from build123d import *

# Parameters (mm, degrees)
SKETCH1_R           = 5
BOSS_EXTRUDE1_DEPTH = 10
SKETCH3_W           = 10
SKETCH3_H           = 4.789047851
BOSS_EXTRUDE2_DEPTH = 15
SKETCH4_W           = 15
SKETCH4_H           = 4.789047851
BOSS_EXTRUDE3_DEPTH = 30
CUT_EXTRUDE1_REACH  = 9.289
SKETCH5_R           = 1.5


with BuildPart() as part:
    # Sketch1 → Boss-Extrude1 (new body)
    with BuildSketch(Plane.XY):
        with BuildLine():
            Line((0, 10), (-35, 7.5))
            Line((-35, 7.5), (-35, -7.5))
            Line((-35, -7.5), (0, -10))
            ThreePointArc((0, -10), (10, 0), (0, 10))
        make_face()
        Circle(SKETCH1_R, mode=Mode.SUBTRACT)
    extrude(amount=BOSS_EXTRUDE1_DEPTH)

    # Sketch3 → Boss-Extrude2 (add)
    with BuildSketch(Plane.ZY.offset(35)):
        with Locations((5, -5.105476075)):
            Rectangle(SKETCH3_W, SKETCH3_H)
    extrude(amount=BOSS_EXTRUDE2_DEPTH)

    # Sketch4 → Boss-Extrude3 (add)
    with BuildSketch(Plane(origin=(0, 0, 0), x_dir=(-1, 0, 0), z_dir=(0, 0, -1))):
        with Locations((42.5, -5.105476075)):
            Rectangle(SKETCH4_W, SKETCH4_H)
    extrude(amount=BOSS_EXTRUDE3_DEPTH)

    # Sketch5 → Cut-Extrude1 (cut, up to next)
    with BuildSketch(Plane(origin=(0, -2.710952149, 0), x_dir=(1, 0, 0), z_dir=(0, 1, 0)), mode=Mode.PRIVATE) as cut_extrude1_sk1:
        with Locations((-39, 2.273461037)):
            Circle(SKETCH5_R)
    cut_extrude1_tool1 = extrude(cut_extrude1_sk1.sketch, amount=-CUT_EXTRUDE1_REACH, mode=Mode.PRIVATE) & part.part
    add(cut_extrude1_tool1.solids().sort_by_distance((-39, -2.710952, -2.273461))[0], mode=Mode.SUBTRACT)
    # Sketch5 → Cut-Extrude1 (cut, up to next)
    with BuildSketch(Plane(origin=(0, -2.710952149, 0), x_dir=(1, 0, 0), z_dir=(0, 1, 0)), mode=Mode.PRIVATE) as cut_extrude1_sk2:
        with Locations((-39, 14.273461037)):
            Circle(SKETCH5_R)
    cut_extrude1_tool2 = extrude(cut_extrude1_sk2.sketch, amount=-CUT_EXTRUDE1_REACH, mode=Mode.PRIVATE) & part.part
    add(cut_extrude1_tool2.solids().sort_by_distance((-39, -2.710952, -14.273461))[0], mode=Mode.SUBTRACT)


solid = part.part
The listing builds one solid part. Answer for the finished solid, in the listing's coordinates (mm). A direction names the side the tool comes from. Round coordinates to 2 decimals unless told otherwise and drop trailing zeros. Write each loop counter-clockwise with the first axis right and the second up, starting at its lowest first coordinate (ties: lowest second). Pieces come first, ordered by that corner, then holes. Notation, with made-up numbers: M -3,-15 L 47,-15 A19 ccw 47,-8 Z; hole C 89,-20.5 d1. An arc over 180 degrees is marked long. Write each question's results on one line, items separated by ' | '. Start each with the question number.
Item 1: Find section A-A on y = 0. Write down the section's boundary in (x, z).
Item 2: Find section B-B on x = -39. Write down the section's boundary in (y, z).
Item 3: Which of the six approach directions +Z, -Z, +X, -X, +Y, -Y give full straight-line access (tool end or side, diameter ignored) to faces 1 (the flat face through (-42, -7.5, -10)), 2 (the flat face through (-35, 2, 5)), 3 (the flat face through (-35, -5, -15))?
Item 4: Straight lines are drawn through the part: probe 1 along Z at (x, y) = (-39, -6.1); probe 2 along X at (y, z) = (-4.25, -20.5); probe 3 along Y at (x, z) = (-45.5, -11). For each, find the intervals that lie inside material, in ascending order.
Item 5: Find section D-D on z = -24. Write down the section's boundary in (x, y), and give its area (3 significant figures).
Item 6: Given pin 1 Ø4 at (y, z) = (-5.5, -10.5) entering from +X; pin 2 Ø1.5 at (x, z) = (-42.5, -25) entering from +Y; pin 3 Ø16.5 at (x, z) = (-41.5, -1) entering from -Y, each flat-ended and moving along its own axis, determine where each tip first touches the part or whether it passes through.
Item 7: Find section C-C on z = 6. Write down the section's boundary in (x, y), and give its area (3 significant figures).
Item 8: The mould has two halves that part along Z. Classify faces 4 (the cylindrical face through (-40.106, -5.072, -15.287)), 5 (the flat face through (-42, -2.711, -10)), 6 (the flat face through (-42, -5, -30)), 7 (the cylindrical face through (-40.19, -5.07, -1.36)): +Z half, -Z half, draft (parallel to the pull), parting line (faces both ways), or undercut.
Answer block:
1) outline: M -35,0 L -5,0 L -5,10 L -35,10 Z; M 5,0 L 10,0 L 10,10 L 5,10 Z
2) outline: M -7.5,-30 L -2.71,-30 L -2.71,-15.77 L -7.5,-15.77 Z; M -7.5,-12.77 L -2.71,-12.77 L -2.71,-3.77 L -7.5,-3.77 Z; M -7.5,-0.77 L -2.71,-0.77 L -2.71,10 L -7.5,10 Z
3) face 1: +Z, -Z, -X, -Y | face 2: +Z, -Z, -X, +Y | face 3: -Z, +X, +Y, -Y
4) probe 1: z = -30 to -15.77, -12.77 to -3.77, -0.77 to 10 | probe 2: x = -50 to -35 | probe 3: y = -7.5 to -2.71
5) outline: M -50,-7.5 L -35,-7.5 L -35,-2.71 L -50,-2.71 Z | area: 71.8 mm²
6) pin 1: stops at x = -35 | pin 2: stops at y = -2.71 | pin 3: stops at y = -7.62
7) outline: M -50,-7.5 L -35,-7.5 L 0,-10 A10 ccw 0,10 L -35,7.5 L -35,-2.71 L -50,-2.71 Z; hole C 0,0 d10 | area: 763 mm²
8) face 4: undercut | face 5: draft | face 6: -Z half | face 7: undercut
